from build123d import *

# Parameters (mm, degrees)
SKETCH_1_R          = 28
EXTRUDE_1_DEPTH     = 2
SKETCH_2_W          = 15
SKETCH_2_H          = 15
EXTRUDE_2_DEPTH     = 1.5
SKETCH_4_W          = 10
SKETCH_4_H          = 20
EXTRUDE_3_DEPTH     = 1.5
SKETCH_5_W          = 15
SKETCH_5_H          = 15
EXTRUDE_4_DEPTH     = 1.5
CUT_EXTRUDE_1_DEPTH = 10


with BuildPart() as part:
    # 草图1 → 凸台-拉伸1 (new body)
    with BuildSketch(Plane.XY):
        Circle(SKETCH_1_R)
    extrude(amount=EXTRUDE_1_DEPTH)

    # 草图2 → 凸台-拉伸2 (add)
    with BuildSketch(Plane.XY.offset(2)):
        Rectangle(SKETCH_2_W, SKETCH_2_H)
    extrude(amount=EXTRUDE_2_DEPTH)

    # 草图4 → 凸台-拉伸3 (add)
    with BuildSketch(Plane(origin=(0, 0, 0), x_dir=(-1, 0, 0), z_dir=(0, 0, -1))):
        with Locations((19, 0)):
            Rectangle(SKETCH_4_W, SKETCH_4_H)
    extrude(amount=EXTRUDE_3_DEPTH)

    # 草图5 → 凸台-拉伸4 (add)
    with BuildSketch(Plane(origin=(0, 0, 0), x_dir=(-1, 0, 0), z_dir=(0, 0, -1))):
        Rectangle(SKETCH_5_W, SKETCH_5_H)
    extrude(amount=EXTRUDE_4_DEPTH)

    # 草图6 → 切除-拉伸1 (cut)
    with BuildSketch(Plane(origin=(0, 0, 0), x_dir=(-1, 0, 0), z_dir=(0, 0, -1))):
        with BuildLine():
            ThreePointArc((-14.495689014, 14.495689014), (-14.495689014, 12.727922061), (-12.727922061, 12.727922061))
            Line((-12.727922061, 12.727922061), (-14.495689014, 14.495689014))
        make_face()
        with BuildLine():
            Line((-14.495689014, 14.495689014), (-12.727922061, 12.727922061))
            ThreePointArc((-12.727922061, 12.727922061), (-12.456956122, 13.133451247), (-12.361805538, 13.611805538))
            ThreePointArc((-12.361805538, 13.611805538), (-13.133451247, 14.766654953), (-14.495689014, 14.495689014))
        make_face()
        with BuildLine():
            ThreePointArc((-12.361805538, -13.611805538), (-12.456956122, -13.133451247), (-12.727922061, -12.727922061))
            Line((-12.727922061, -12.727922061), (-14.495689014, -14.495689014))
            ThreePointArc((-14.495689014, -14.495689014), (-13.133451247, -14.766654953), (-12.361805538, -13.611805538))
        make_face()
        with BuildLine():
            Line((-14.495689014, -14.495689014), (-12.727922061, -12.727922061))
            ThreePointArc((-12.727922061, -12.727922061), (-14.495689014, -12.727922061), (-14.495689014, -14.495689014))
        make_face()
        with BuildLine():
            ThreePointArc((14.861805538, -13.611805538), (14.090159828, -12.456956122), (12.727922061, -12.727922061))
            Line((12.727922061, -12.727922061), (14.495689014, -14.495689014))
            ThreePointArc((14.495689014, -14.495689014), (14.766654953, -14.090159828), (14.861805538, -13.611805538))
        make_face()
        with BuildLine():
            Line((14.495689014, -14.495689014), (12.727922061, -12.727922061))
            ThreePointArc((12.727922061, -12.727922061), (12.727922061, -14.495689014), (14.495689014, -14.495689014))
        make_face()
        with BuildLine():
            ThreePointArc((14.495689014, 14.495689014), (12.727922061, 14.495689014), (12.727922061, 12.727922061))
            Line((12.727922061, 12.727922061), (14.495689014, 14.495689014))
        make_face()
        with BuildLine():
            Line((14.495689014, 14.495689014), (12.727922061, 12.727922061))
            ThreePointArc((12.727922061, 12.727922061), (14.090159828, 12.456956122), (14.861805538, 13.611805538))
            ThreePointArc((14.861805538, 13.611805538), (14.766654953, 14.090159828), (14.495689014, 14.495689014))
        make_face()
    extrude(amount=-CUT_EXTRUDE_1_DEPTH, mode=Mode.SUBTRACT)


solid = part.part
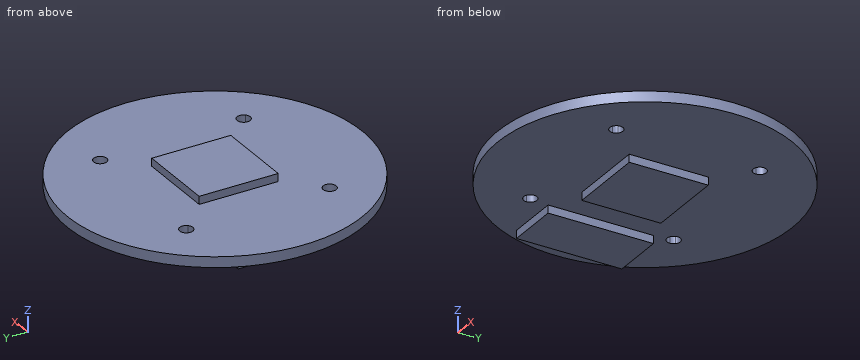
Can you work these out from the model? Positions are in its coordinate system, mm. Round coordinates to 2 decimals unless told otherwise and drop trailing zeros. Order: outer loops, then holes, each group sorted by start corner. A loop starts at its lowest first (then second) coordinate and runs counter-clockwise, first axis right, second up. Notation, with made-up numbers: (47, 59) - (87, 59) arc R27 ccw to (87, 93) - close; hole circle Ø8 at (18, 62.5). An arc over 180 degrees is marked (long way). Answer in a Markdown table with one row per item.
(1) Suppose I cut it at C-C, the plane x = 19.5. Please give me the cut outline in (y, z), plus the area to 3 significant figures.
From the geometry:
| item | result |
|---|---|
| outline | (-20.09, 0) - (20.09, 0) - (20.09, 2) - (-20.09, 2) - close |
| area | 80.4 mm2 |
(2) Please list where these lines run through material, in increasing order: L1, parallel to X at y = -5.5, z = -0.7; L2, parallel to X at y = 13.5, z = 0.15; L3, parallel to Y at x = 3, z = 3.1. Write a range as from..to.
From the geometry:
| item | result |
|---|---|
| L1 | x = -24..-14, -7.5..7.5 |
| L2 | x = -24.53..-14.86, -12.37..12.37, 14.86..24.53 |
| L3 | y = -7.5..7.5 |
(3) Suppose I cut it at A-A, the plane y = 0. Please give me the cut outline in (x, z).
From the geometry:
| item | result |
|---|---|
| outline | (-28, 0) - (-24, 0) - (-24, -1.5) - (-14, -1.5) - (-14, 0) - (-7.5, 0) - (-7.5, -1.5) - (7.5, -1.5) - (7.5, 0) - (28, 0) - (28, 2) - (7.5, 2) - (7.5, 3.5) - (-7.5, 3.5) - (-7.5, 2) - (-28, 2) - close |
(4) For P1, Ø1.6, axis at y = -0.5, z = -0.5, coming from the +X side; P2, Ø3, axis at x = 7.5, z = 2, coming from the -Y side; P3, Ø2, axis at y = -18.5, z = 2.5, coming from the +X side; P4, Ø0.8, axis at x = -2.5, z = -0.5, coming from the +Y side, each with a flat end and sliding along its axis, tell me the tip position at first contact or that it passes through.
From the geometry:
| item | result |
|---|---|
| P1 | stops at x = 28 |
| P2 | stops at y = -27.35 |
| P3 | stops at x = 21.75 |
| P4 | stops at y = 7.5 |
(5) Suppose I cut it at B-B, the plane x = 0. Please give me the cut outline in (y, z), plus the area to 3 significant figures.
From the geometry:
| item | result |
|---|---|
| outline | (-28, 0) - (-7.5, 0) - (-7.5, -1.5) - (7.5, -1.5) - (7.5, 0) - (28, 0) - (28, 2) - (7.5, 2) - (7.5, 3.5) - (-7.5, 3.5) - (-7.5, 2) - (-28, 2) - close |
| area | 157 mm2 |
